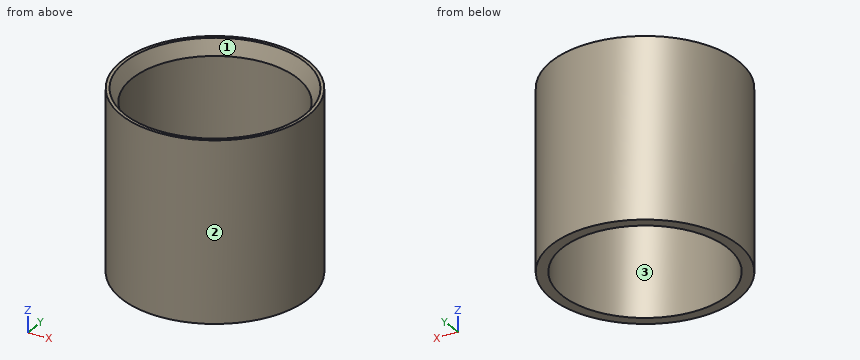
```python
from build123d import *

# Parameters (mm, degrees)
F0_R     = 17.4371
F0_R_2   = 16.8275
F0_R_3   = 15.4305
F1_DEPTH = 31.6992
F2_DEPTH = 1.6383
F3_SIZE2 = 1.4079449907
F3_SIZE  = 2.54


with BuildPart() as f1:
    # F0 (on Top) → F1 (new body)
    with BuildSketch(Plane.XY):
        Circle(F0_R)
        Circle(F0_R_2, mode=Mode.SUBTRACT)
        Circle(F0_R_2)
        Circle(F0_R_3, mode=Mode.SUBTRACT)
    extrude(amount=F1_DEPTH)

    # F0 (on Top) → F2 (join)
    with BuildSketch(Plane.XY):
        Circle(F0_R)
        Circle(F0_R_2, mode=Mode.SUBTRACT)
        Circle(F0_R_2)
        Circle(F0_R_3, mode=Mode.SUBTRACT)
    extrude(amount=-F2_DEPTH)

    # F3
    f3_edges = [f1.edges().sort_by_distance(p)[0] for p in [
        (-15.4305, 0, 31.6992),
    ]]
    f3_side = f1.faces().sort_by_distance((-15.4305, 0, 15.8496))[0]
    chamfer(f3_edges, length=F3_SIZE, length2=F3_SIZE2, reference=f3_side)


solid = f1.part
```
Could you check a few things on this model? Use its own coordinates, in mm. Face numbers are marked on the shaded views. Coordinates: 2 decimals unless noted, no trailing zeros. Loops run counter-clockwise (first coordinate to the right, second up) from the corner with the lowest first, then second, coordinate; pieces in that order, holes last.
1) Will these pins go through, and if not, where does the flat tip stop? pin 1 Ø1.5 at (x, z) = (13.5, 25) entering from +Y; pin 2 Ø1 at (y, z) = (7.5, 16.5) entering from -X; pin 3 Ø12 at (x, z) = (-12.5, 13.5) entering from -Y.
Reported:
pin 1: stops at y = 11.89
pin 2: stops at x = -15.97
pin 3: stops at y = -16.18
2) Thinking about a two-plate mould opening in X: for the marked faces 1, 2 and 3, which applies, released by +X, released by -X, zero draft, split by the parting line, or undercut?
Reported:
face 1: undercut
face 2: split by the parting line
face 3: undercut
3) Imagine slicing it at C-C (z = 28). List the corners of the cut face in (x, y) for me, and give its area (3 significant figures).
Reported:
outline: circle Ø34.87 at (0, 0); hole circle Ø30.86 at (0, 0)
area: 207 mm2
4) Imagine slicing it at A-A (x = 0). List the corners of the cut face in (y, z) for me.
Reported:
outline: (-17.44, -1.64) - (-15.43, -1.64) - (-15.43, 29.16) - (-16.84, 31.7) - (-17.44, 31.7) - close; (15.43, -1.64) - (17.44, -1.64) - (17.44, 31.7) - (16.84, 31.7) - (15.43, 29.16) - close
5) Please list where these lines run through material, in increasing order: line 1 along Y through (x, z) = (0, 21.5); line 2 along X through (y, z) = (-12, 26.5); line 3 along X through (y, z) = (10.5, 21.5).
Reported:
line 1: y = -17.44 to -15.43, 15.43 to 17.44
line 2: x = -12.65 to -9.7, 9.7 to 12.65
line 3: x = -13.92 to -11.31, 11.31 to 13.92
